from build123d import *

# Parameters (mm, degrees)
SKETCH1_W           = 120
SKETCH1_H           = 42.16
BOSS_EXTRUDE1_DEPTH = 21
CUT_EXTRUDE1_DEPTH  = 14
SKETCH3_R           = 3.25
CUT_EXTRUDE2_DEPTH  = 82.007752785
FILLET1_R           = 1
FILLET2_R           = 0.5
BOSS_EXTRUDE2_DEPTH = 53


with BuildPart() as part:
    # Sketch1 → Boss-Extrude1 (new body)
    with BuildSketch(Plane(origin=(0, 0, 0), x_dir=(1, 0, 0), z_dir=(0, 1, 0))):
        with Locations((16.811029237, -0.514485382)):
            Rectangle(SKETCH1_W, SKETCH1_H)
    extrude(amount=BOSS_EXTRUDE1_DEPTH)

    # Sketch2 → Cut-Extrude1 (cut)
    with BuildSketch(Plane(origin=(0, 21, 0), x_dir=(1, 0, 0), z_dir=(0, 1, 0))):
        with BuildLine():
            ThreePointArc((27.061029237, 5.735514618), (20.811029237, -0.514485382), (27.061029237, -6.764485382))
            Line((27.061029237, -6.764485382), (27.061029237, 5.735514618))
        make_face()
        with BuildLine():
            Line((27.061029237, 5.735514618), (27.061029237, -6.764485382))
            ThreePointArc((27.061029237, -6.764485382), (31.480446619, -4.933902764), (33.311029237, -0.514485382))
            ThreePointArc((33.311029237, -0.514485382), (31.480446619, 3.904932001), (27.061029237, 5.735514618))
        make_face()
        with BuildLine():
            ThreePointArc((6.561029237, 5.735514618), (0.311029237, -0.514485382), (6.561029237, -6.764485382))
            Line((6.561029237, -6.764485382), (6.561029237, 5.735514618))
        make_face()
        with BuildLine():
            Line((6.561029237, 5.735514618), (6.561029237, -6.764485382))
            ThreePointArc((6.561029237, -6.764485382), (10.980446619, -4.933902764), (12.811029237, -0.514485382))
            ThreePointArc((12.811029237, -0.514485382), (10.980446619, 3.904932001), (6.561029237, 5.735514618))
        make_face()
    extrude(amount=-CUT_EXTRUDE1_DEPTH, mode=Mode.SUBTRACT)

    # Sketch3 → Cut-Extrude2 (cut, through all)
    with BuildSketch(Plane(origin=(0, 7, 0), x_dir=(1, 0, 0), z_dir=(0, 1, 0))):
        with Locations(Location((27.061029237, -0.514485382, 0), (0, 0, 270))):
            Circle(SKETCH3_R)
        with Locations(Location((6.561029237, -0.514485382, 0), (0, 0, 270))):
            Circle(SKETCH3_R)
    extrude(amount=-CUT_EXTRUDE2_DEPTH, mode=Mode.SUBTRACT)

    # Fillet1
    fillet1_edges = [part.edges().sort_by_distance(p)[0] for p in [
        (27.061029237, 21, 6.764485382),
        (6.561029237, 21, 6.764485382),
    ]]
    fillet(fillet1_edges, radius=FILLET1_R)

    # Fillet2
    fillet2_edges = [part.edges().sort_by_distance(p)[0] for p in [
        (27.061029237, 0, -2.735514618),
        (6.561029237, 0, -2.735514618),
    ]]
    fillet(fillet2_edges, radius=FILLET2_R)

    # Sketch4 → Boss-Extrude2 (add)
    with BuildSketch(Plane(origin=(0, 21, 0), x_dir=(1, 0, 0), z_dir=(0, 1, 0))):
        with BuildLine():
            ThreePointArc((52.461029237, 3.485514618), (48.461029237, -0.514485382), (52.461029237, -4.514485382))
            Line((52.461029237, -4.514485382), (52.461029237, 3.485514618))
        make_face()
        with BuildLine():
            Line((52.461029237, 3.485514618), (52.461029237, -4.514485382))
            ThreePointArc((52.461029237, -4.514485382), (55.289456362, -3.342912506), (56.461029237, -0.514485382))
            ThreePointArc((56.461029237, -0.514485382), (55.289456362, 2.313941743), (52.461029237, 3.485514618))
        make_face()
        with BuildLine():
            ThreePointArc((-18.838970763, 3.485514618), (-22.838970763, -0.514485382), (-18.838970763, -4.514485382))
            Line((-18.838970763, -4.514485382), (-18.838970763, 3.485514618))
        make_face()
        with BuildLine():
            Line((-18.838970763, 3.485514618), (-18.838970763, -4.514485382))
            ThreePointArc((-18.838970763, -4.514485382), (-16.010543638, -3.342912506), (-14.838970763, -0.514485382))
            ThreePointArc((-14.838970763, -0.514485382), (-16.010543638, 2.313941743), (-18.838970763, 3.485514618))
        make_face()
    extrude(amount=BOSS_EXTRUDE2_DEPTH)


solid = part.part
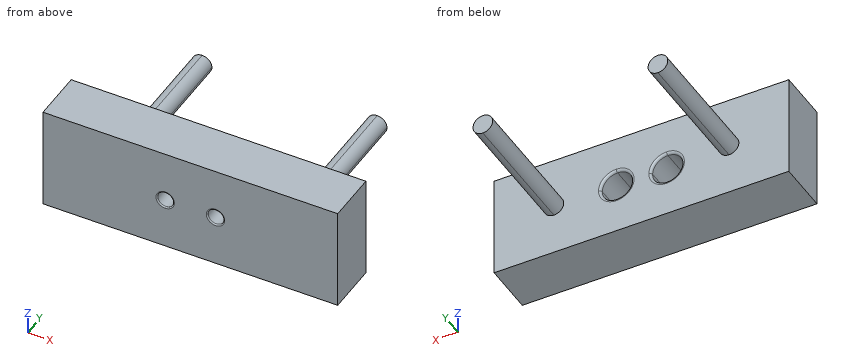
The model under review builds one solid part; all positions refer to its coordinate system, in mm. Round coordinates to 2 decimals unless told otherwise and drop trailing zeros. Write each loop counter-clockwise with the first axis right and the second up, starting at its lowest first coordinate (ties: lowest second). Pieces come first, ordered by that corner, then holes. Notation, with made-up numbers: (44, 49) - (62, 49) arc R13 ccw to (62, 68) - close; hole circle Ø11 at (-3.75, 46). An arc over 180 degrees is marked (long way). One line per item, written item: value. Start each with the question number.
1. Consider section C-C on x = 50.5. Write out the cut boundary in (y, z).
2. Clearance check with flat-ended pins moving along their axes: P1, Ø14, axis at x = 25.5, z = -0.5, coming from the +Y side; P2, Ø10, axis at x = 26, z = 1, coming from the -Y side; P3, Ø6, axis at x = 27.06, z = 0.51, coming from the -Y side; P4, Ø7.5, axis at x = 6.56, z = 0.51, coming from the +Y side. State where each tip first meets the part, or that it passes through.
3. Consider section A-A on y = 49. Write out the cut boundary in (x, z), and give its area (3 significant figures).
4. Consider section D-D on z = -11. Write out the cut boundary in (x, y).
5. To check wall thickness, follow L1, parallel to Y at x = -13, z = -7.5; L2, parallel to X at y = 36.5, z = 2.5; L3, parallel to X at y = 38, z = 3. State the ranges of each line that lie inside material, in increasing order. Write a range as from..to.
6. Consider section B-B on y = 11.5. Write out the cut boundary in (x, z), and give its area (3 significant figures).
Checks:
1. outline: (0, -20.57) - (21, -20.57) - (21, -2.97) - (74, -2.97) - (74, 4) - (21, 4) - (21, 21.59) - (0, 21.59) - close
2. P1: stops at y = 21
2. P2: stops at y = 0
2. P3: passes through
2. P4: stops at y = 7
3. outline: circle Ø8 at (-18.84, 0.51); circle Ø8 at (52.46, 0.51)
3. area: 101 mm^2
4. outline: (-43.19, 0) - (76.81, 0) - (76.81, 21) - (-43.19, 21) - close
5. L1: y = 0..21
5. L2: x = -22.31..-15.37, 48.99..55.93
5. L3: x = -21.97..-15.7, 49.33..55.6
6. outline: (-43.19, -20.57) - (76.81, -20.57) - (76.81, 21.59) - (-43.19, 21.59) - close; hole circle Ø12.5 at (6.56, 0.51); hole circle Ø12.5 at (27.06, 0.51)
6. area: 4,810 mm^2
